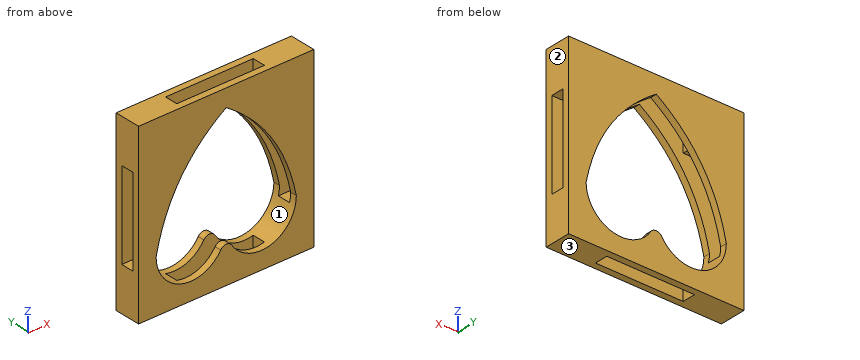
```python
from build123d import *

# Parameters (mm, degrees)
SKETCH1_W           = 20
SKETCH1_H           = 20
BOSS_EXTRUDE1_DEPTH = 3
SKETCH2_W           = 10
SKETCH2_H           = 1.5
CUT_EXTRUDE1_DEPTH  = 21.0000001
SKETCH3_W           = 10
SKETCH3_H           = 1.5
CUT_EXTRUDE2_DEPTH  = 21.0000001


with BuildPart() as part:
    # Sketch1 → Boss-Extrude1 (new body)
    with BuildSketch(Plane(origin=(0, 0, 0), x_dir=(1, 0, 0), z_dir=(0, 1, 0))):
        Rectangle(SKETCH1_W, SKETCH1_H)
        with BuildLine():
            ThreePointArc((-0.631578947, 6.157252793), (-5.123902974, 7.83885948), (-8, 4))
            add(Edge.make_bspline(
                [(-8, 4), (-6.403336947, -3.811544104), (0, -8)],
                knots=[0, 0, 0, 1, 1, 1], degree=2))
            add(Edge.make_bspline(
                [(8, 4), (6.403336947, -3.811544104), (0, -8)],
                knots=[0, 0, 0, 1, 1, 1], degree=2))
            ThreePointArc((8, 4), (5.123902974, 7.83885948), (0.631578947, 6.157252793))
            ThreePointArc((0.631578947, 6.157252793), (0, 5.811737691), (-0.631578947, 6.157252793))
        make_face(mode=Mode.SUBTRACT)
    extrude(amount=BOSS_EXTRUDE1_DEPTH)

    # Sketch2 → Cut-Extrude1 (cut, through all)
    with BuildSketch(Plane(origin=(10, 0, 0), x_dir=(0, 0, -1), z_dir=(1, 0, 0))):
        with Locations((0, 1.5)):
            Rectangle(SKETCH2_W, SKETCH2_H)
    extrude(amount=-CUT_EXTRUDE1_DEPTH, mode=Mode.SUBTRACT)

    # Sketch3 → Cut-Extrude2 (cut, through all)
    with BuildSketch(Plane.XY.offset(10)):
        with Locations((0, 1.5)):
            Rectangle(SKETCH3_W, SKETCH3_H)
    extrude(amount=-CUT_EXTRUDE2_DEPTH, mode=Mode.SUBTRACT)


solid = part.part
```
Model file for the job. Use its own axes, mm. Face numbers are marked on the shaded views. Round coordinates to 2 decimals unless told otherwise and drop trailing zeros. Write each loop counter-clockwise with the first axis right and the second up, starting at its lowest first coordinate (ties: lowest second). Pieces come first, ordered by that corner, then holes. Notation, with made-up numbers: M 66.25,3.25 L 114.25,3.25 A17 ccw 114.25,28.25 Z; hole C 68.5,-27 d9. An arc over 180 degrees is marked long. Put each result on its own line as item: value.
Item 1: Probe L1, parallel to Y at x = 8.5, z = 2.5; L2, parallel to X at y = 2, z = 6.5. List the from-to ranges inside material, lowest first. Write a range as from..to.
Responses:
L1: 0..0.75, 2.25..3
L2: -10..-5, 5..10
Item 2: Mould opens along Z. For the marked faces 1, 2 and 3 say: +Z half, -Z half, draft (parallel to the pull), parting line (faces both ways), or undercut.
Responses:
face 1: undercut
face 2: draft
face 3: -Z half
Item 3: Cut at B-B (x = -2.5). State how many separate pieces and enclosed holes the cut face has, and give its area (3 significant figures).
Responses:
separate pieces: 4
enclosed holes: 0
area: 9.35 mm²
Item 4: Cut at A-A (y = 1.2). List the corners of the cut face in (x, z), and give its area (3 significant figures).
Responses:
outline: M -10,-10 L -5,-10 L -5,-7.87 A4 cw -7.87,-5 L -10,-5 Z; M -10,5 L -5,5 L -5,10 L -10,10 Z; M 5,-10 L 10,-10 L 10,-5 L 7.87,-5 A4 cw 5,-7.87 Z; M 5,5 L 10,5 L 10,10 L 5,10 Z
area: 88.7 mm²
